```python
from build123d import *

# Parameters (mm, degrees)
SKETCH1_W           = 111
SKETCH1_H           = 60
BOSS_EXTRUDE1_DEPTH = 2
SKETCH2_R           = 10
SKETCH2_R_2         = 1
SKETCH2_R_3         = 2.5
CUT_EXTRUDE1_DEPTH  = 3
FILLET1_R           = 2.5
FILLET2_R           = 1


with BuildPart() as part:
    # Sketch1 → Boss-Extrude1 (new body)
    with BuildSketch(Plane(origin=(0, 0, 0), x_dir=(1, 0, 0), z_dir=(0, 1, 0))):
        with Locations((55.5, 30)):
            Rectangle(SKETCH1_W, SKETCH1_H)
    extrude(amount=BOSS_EXTRUDE1_DEPTH)

    # Sketch2 → Cut-Extrude1 (cut, through all)
    with BuildSketch(Plane(origin=(0, 2, 0), x_dir=(1, 0, 0), z_dir=(0, 1, 0))):
        with Locations((87.735933435, 22.928451884)):
            Circle(SKETCH2_R)
        with Locations((2.5, 57.5)):
            Circle(SKETCH2_R_2)
        with Locations((108.5, 57.5)):
            Circle(SKETCH2_R_2)
        with Locations((108.5, 2.5)):
            Circle(SKETCH2_R_2)
        with Locations((2.5, 2.5)):
            Circle(SKETCH2_R_2)
        with Locations((25.9625, 30)):
            Circle(SKETCH2_R_3)
        with Locations((25.9625, 40.118198487)):
            Circle(SKETCH2_R_3)
    extrude(amount=-CUT_EXTRUDE1_DEPTH, mode=Mode.SUBTRACT)

    # Fillet1
    fillet1_edges = [part.edges().sort_by_distance(p)[0] for p in [
        (0, 1, -60),
        (111, 1, -60),
        (111, 1, 0),
        (0, 1, 0),
    ]]
    fillet(fillet1_edges, radius=FILLET1_R)

    # Fillet2
    fillet2_edges = [part.edges().sort_by_distance(p)[0] for p in [
        (0, 2, -30),
        (55.5, 2, -60),
        (55.5, 2, 0),
        (111, 2, -30),
        (110.267766953, 2, -0.732233047),
        (110.267766953, 2, -59.267766953),
        (0.732233047, 2, -0.732233047),
        (0.732233047, 2, -59.267766953),
    ]]
    fillet(fillet2_edges, radius=FILLET2_R)


solid = part.part
```
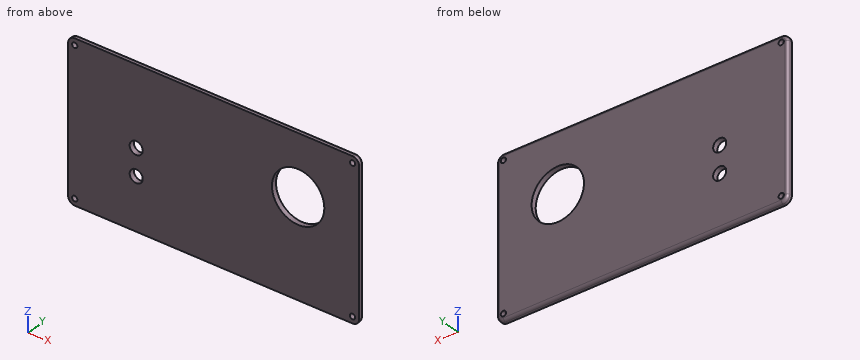
Could you check a few things on this model? Use its own coordinates, in mm. Give positions to 0.01 mm unless a question says otherwise; leave off trailing zeros. Order: outer loops, then holes, each group sorted by start corner. A loop starts at its lowest first (then second) coordinate and runs counter-clockwise, first axis right, second up.
Q1. Suppose I cut it at C-C, the plane z = -18. Write out the boundary of the cut face in (x, y), and give its area (3 significant figures).
Q2. Suppose I cut it at B-B, the plane y = 1.4. Write out the boundary of the cut face in (x, z), and give its area (3 significant figures).
Q3. If I drill on line 1 along Z through (x, y) = (108.5, 1.05); line 2 along X through (y, z) = (1.05, -57.5); line 3 along Z through (x, y) = (26.5, 1), over which ranges is the centre line in solid material (lowest first)?
Q4. Suppose I cut it at A-A, the plane z = -30. Write out the boundary of the cut face in (x, y).
Solution:
1. outline: (0, 0) - (79.03, 0) - (79.03, 2) - (1, 2) arc R1 ccw to (0, 1) - close; (96.44, 0) - (111, 0) - (111, 1) arc R1 ccw to (110, 2) - (96.44, 2) - close
1. area: 187 mm2
2. outline: (0.08, -57.5) arc R2.42 ccw to (2.5, -59.92) - (108.5, -59.92) arc R2.42 ccw to (110.92, -57.5) - (110.92, -2.5) arc R2.42 ccw to (108.5, -0.08) - (2.5, -0.08) arc R2.42 ccw to (0.08, -2.5) - close; hole circle Ø2 at (2.5, -57.5); hole circle Ø2 at (2.5, -2.5); hole circle Ø5 at (25.96, -40.12); hole circle Ø5 at (25.96, -30); hole circle Ø20 at (87.74, -22.93); hole circle Ø2 at (108.5, -57.5); hole circle Ø2 at (108.5, -2.5)
2. area: 6,260 mm2
3. line 1: z = -60 to -58.5, -56.5 to -3.5, -1.5 to 0
3. line 2: x = 0 to 1.5, 3.5 to 107.5, 109.5 to 111
3. line 3: z = -60 to -42.56, -37.68 to -32.44, -27.56 to 0
4. outline: (0, 0) - (23.46, 0) - (23.46, 2) - (1, 2) arc R1 ccw to (0, 1) - close; (28.46, 0) - (80.67, 0) - (80.67, 2) - (28.46, 2) - close; (94.81, 0) - (111, 0) - (111, 1) arc R1 ccw to (110, 2) - (94.81, 2) - close
